from build123d import *

# Parameters (mm, degrees)
PAD_DEPTH              = 13.4
CYLINDER_W             = 6.7
CYLINDER_H             = 298.45
CYLINDER_ANGLE         = 180
CYLINDER001_R          = 99.483333
CYLINDER001_DEPTH      = 32
BOX_W                  = 149.225
BOX_H                  = 30
BOX_DEPTH              = 21
BOX001_W               = 33
BOX001_H               = 149.225
BOX001_DEPTH           = 22
CYLINDER002_R          = 3.7
CYLINDER002_DEPTH      = 105
LINEARPATTERN_COUNT    = 3
LINEARPATTERN_PITCH    = 74.6125
CYLINDER003_R          = 1.85
CYLINDER003_DEPTH      = 100
LINEARPATTERN001_COUNT = 3
LINEARPATTERN001_PITCH = 74.6125
CYLINDER004_R          = 2.55
CYLINDER004_DEPTH      = 10
LINEARPATTERN002_COUNT = 3
LINEARPATTERN002_PITCH = 141.16875


with BuildPart() as part:
    # Sketch → Pad (new body)
    with BuildSketch(Plane.XY):
        Polygon((0, 0), (298.45, 0), (0, 298.45), align=None)
    extrude(amount=PAD_DEPTH)

    # Cylinder → Cylinder (revolve, cut)
    with BuildSketch(Plane(origin=(0, 0, 6.7), x_dir=(0, 0, 1), z_dir=(-1, 0, 0))):
        with Locations((3.35, 149.225)):
            Rectangle(CYLINDER_W, CYLINDER_H)
    revolve(axis=Axis((0, 0, 6.7), (0, 1, 0)), revolution_arc=CYLINDER_ANGLE, mode=Mode.SUBTRACT)

    # Cylinder001 → Cylinder001 (cut)
    with BuildSketch(Plane(origin=(149.225, 149.225, -8), x_dir=(1, 0, 0), z_dir=(0, 0, 1))):
        Circle(CYLINDER001_R)
    extrude(amount=CYLINDER001_DEPTH, mode=Mode.SUBTRACT)

    # Box → Box (cut)
    with BuildSketch(Plane(origin=(149.225, 79.741667, 17), x_dir=(1, 0, 0), z_dir=(0, 0, -1))):
        with Locations((74.6125, 15)):
            Rectangle(BOX_W, BOX_H)
    extrude(amount=BOX_DEPTH, mode=Mode.SUBTRACT)

    # Box001 → Box001 (cut)
    with BuildSketch(Plane(origin=(49.741667, 303.579167, 17), x_dir=(1, 0, 0), z_dir=(0, 0, -1))):
        with Locations((16.5, 74.6125)):
            Rectangle(BOX001_W, BOX001_H)
    extrude(amount=BOX001_DEPTH, mode=Mode.SUBTRACT)

    # Cylinder002 → Cylinder002 (cut)
    with BuildSketch(Plane(origin=(74.6125, 5, 6.7), x_dir=(-1, 0, 0), z_dir=(0, 1, 0))):
        Circle(CYLINDER002_R)
    cylinder002 = extrude(amount=CYLINDER002_DEPTH, mode=Mode.SUBTRACT)

    # LinearPattern: Cylinder002 ×3
    with Locations(*[(i * LINEARPATTERN_PITCH, 0, 0) for i in range(1, LINEARPATTERN_COUNT)]):
        add(cylinder002, mode=Mode.SUBTRACT)

    # Cylinder003 → Cylinder003 (cut)
    with BuildSketch(Plane(origin=(74.6125, 0, 6.7), x_dir=(-1, 0, 0), z_dir=(0, 1, 0))):
        Circle(CYLINDER003_R)
    cylinder003 = extrude(amount=CYLINDER003_DEPTH, mode=Mode.SUBTRACT)

    # LinearPattern001: Cylinder003 ×3
    with Locations(*[(i * LINEARPATTERN001_PITCH, 0, 0) for i in range(1, LINEARPATTERN001_COUNT)]):
        add(cylinder003, mode=Mode.SUBTRACT)

    # Cylinder004 → Cylinder004 (cut)
    with BuildSketch(Plane(origin=(0, 8.05625, 0), x_dir=(1, 0, 0), z_dir=(0, 0, 1))):
        Circle(CYLINDER004_R)
    cylinder004 = extrude(amount=CYLINDER004_DEPTH, mode=Mode.SUBTRACT)

    # LinearPattern002: Cylinder004 ×3
    with Locations(*[(0, i * LINEARPATTERN002_PITCH, 0) for i in range(1, LINEARPATTERN002_COUNT)]):
        add(cylinder004, mode=Mode.SUBTRACT)


solid = part.part
Work out the finished part from the listing and answer in its coordinate system (mm). A direction names the side the tool comes from. Coordinates: 2 decimals unless noted, no trailing zeros. Write each loop counter-clockwise with the first axis right and the second up, starting at its lowest first coordinate (ties: lowest second). Pieces come first, ordered by that corner, then holes. Notation, with made-up numbers: (-25, -32) - (2, -32) arc R10 cw to (2, -20) - close; hole circle Ø5 at (-14, 75.5). An arc over 180 degrees is marked (long way). One line per question, with ' | ' between items.
1) Find section A-A, the plane y = 19. Give the number of separate pieces and of enclosed holes in the cut face, and give its area (3 significant figures).
Checks:
separate pieces: 1 | enclosed holes: 3 | area: 3,550 mm2
2) Flat-ended cylindrical pins translate along their axes: P1, Ø4.5, axis at x = 74.61, z = 6.7, coming from the +Y side; P2, Ø3, axis at y = 150, z = 9.5, coming from the +X side; P3, Ø2, axis at y = 204, z = 6, coming from the -X side. Find the tip coordinate at first contact, or state that the pin passes through.
Checks:
P1: y = 5 | P2: x = 49.77 | P3: x = 6.48
3) For faces 1 (the face through (49.742, 202, 7)), 2 (the face through (6.7, 151.3, 6.8)), 3 (the face through (73, 5, 5)), determine the directions among +Z, -Z, +X, -X, +Y, -Y from which every point of the face is accessible in a straight line to the end or side of a thin tool.
Checks:
face 1: +Z, -Z, +X, +Y | face 2: -X, +Y, -Y | face 3: +Y
4) Find section B-B, the plane x = 235. Determine the outline of the cut face in (y, z), and give its area (3 significant figures).
Checks:
outline: (0, 0) - (49.74, 0) - (49.74, 13.4) - (0, 13.4) - close | area: 667 mm2
5) Consider probe 1 along X at (y, z) = (14, 8.5); probe 2 along X at (y, z) = (23, 6.5); probe 3 along Y at (x, z) = (152.5, 12). Determine where each line is inside the solid, lowest interval first. Write a range as [from, to].
Checks:
probe 1: [6.45, 71.38], [77.85, 145.99], [152.46, 220.6], [227.07, 284.45] | probe 2: [6.7, 70.92], [78.31, 145.53], [152.92, 220.14], [227.53, 275.45] | probe 3: [0, 49.74]
6) Find section C-C, the plane y = 184. Determine the outline of the cut face in (x, z).
Checks:
outline: (0, 0) - (49.74, 0) - (49.74, 13.4) - (0, 13.4) arc R6.7 cw to start
7) The mould has two halves that part along Z. Classify faces 4 (the face through (60, 84, 13.4)), 5 (the face through (71.083, 45.856, 7.811)), 6 (the face through (147, 0, 7)): +Z half, -Z half, draft (parallel to the pull), parting line (faces both ways), or undercut.
Checks:
face 4: +Z half | face 5: undercut | face 6: draft
